from build123d import *

# Parameters (mm, degrees)
F1_DEPTH = 1.8542
F2_W     = 1.143
F2_H     = 2.4384
F3_DEPTH = 25.4


with BuildPart() as f1:
    # F0 (on Front) → F1 (new body, symmetric)
    with BuildSketch(Plane.XZ):
        Polygon((-6.975146, 2.699733), (-0.1143, 0), (-0.1143, -16.9164), (0.290897, -18.905481), (0.514896, -18.85985), (0.1143, -16.9164), (0.1143, 0), (0.1143, 0.155708), (-6.89144, 2.912456), align=None)
    extrude(amount=F1_DEPTH, both=True)

    # F2 (on face) → F3 (cut)
    with BuildSketch(Plane(origin=(-0.1143, 0, 0), x_dir=(0, -1, 0), z_dir=(-1, 0, 0))):
        with BuildLine():
            Line((-1.8542, -11.176), (-1.8542, -8.636))
            ThreePointArc((-1.8542, -8.636), (-3.1242, -9.906), (-1.8542, -11.176))
        make_face()
        with BuildLine():
            ThreePointArc((-0.5842, -9.906), (-0.956174, -9.007974), (-1.8542, -8.636))
            Line((-1.8542, -8.636), (-1.8542, -11.176))
            ThreePointArc((-1.8542, -11.176), (-0.956174, -10.804026), (-0.5842, -9.906))
        make_face()
        with BuildLine():
            ThreePointArc((3.1242, -9.906), (2.752226, -9.007974), (1.8542, -8.636))
            Line((1.8542, -8.636), (1.8542, -11.176))
            ThreePointArc((1.8542, -11.176), (2.752226, -10.804026), (3.1242, -9.906))
        make_face()
        with BuildLine():
            Line((1.8542, -11.176), (1.8542, -8.636))
            ThreePointArc((1.8542, -8.636), (0.5842, -9.906), (1.8542, -11.176))
        make_face()
        with Locations((-1.2827, -3.7592)):
            Rectangle(F2_W, F2_H)
    extrude(amount=-F3_DEPTH, mode=Mode.SUBTRACT)


solid = f1.part
Geometry: final body of the model. Coordinates: model frame, mm. A direction names the side the tool comes from. Give positions to 0.01 mm unless a question says otherwise; leave off trailing zeros. Order: outer loops, then holes, each group sorted by start corner. A loop starts at its lowest first (then second) coordinate and runs counter-clockwise, first axis right, second up. Notation, with made-up numbers: (27, 28) - (71, 28) arc R36 ccw to (71, 66) - close; hole circle Ø4 at (-29.75, -24.5). An arc over 180 degrees is marked (long way). Use CSV: the item, a comma, the result in double quotes.
1. Contact query for flat-ended pins moving along their axis: pin 1 (1.5 mm diameter, centred on x = -4, y = 0, fed in from +Z); pin 2 (1.1 mm diameter, centred on y = -0.5, z = -9, fed in from +X). Output: stop coordinate, or through.
Answers below:
pin 1,"z = 2.07"
pin 2,"x = 0.11"
2. Material intervals for line 1 along X through (y, z) = (0.75, -8.5); line 2 along Z through (x, y) = (-4.5, 1.45); line 3 along Z through (x, y) = (-6, 1.4), sorted ascending. Write a range as from..to.
Answers below:
line 1,"-0.11..0.11"
line 2,"1.73..1.97"
line 3,"2.32..2.56"
3. Section query A-A (y = -1.55). Output: boundary loops of the cut face in (x, z), plus the area to 3 significant figures.
Answers below:
outline,"(-6.98, 2.7) - (-0.11, 0) - (-0.11, -8.67) - (0.11, -8.67) - (0.11, 0.16) - (-6.89, 2.91) - close; (-0.11, -16.92) - (0.29, -18.91) - (0.51, -18.86) - (0.11, -16.92) - (0.11, -11.14) - (-0.11, -11.14) - close"
area,"5.48 mm2"
4. Section query B-B (y = 0.3). Output: boundary loops of the cut face in (x, z), plus the area to 3 significant figures.
Answers below:
outline,"(-6.98, 2.7) - (-0.11, 0) - (-0.11, -16.92) - (0.29, -18.91) - (0.51, -18.86) - (0.11, -16.92) - (0.11, 0.16) - (-6.89, 2.91) - close"
area,"6.04 mm2"
5. Access query for faces 1 (the face through (0.114, 0, -8)), 2 (the face through (-0.114, 0, -8)). Directions: +Z, -Z, +X, -X, +Y, -Y. A direction counts if a zero-diameter tool reaches every point of the face in a straight line with its end or side. Return the directions, or none.
Answers below:
face 1,"+Z, +X, +Y, -Y"
face 2,"-Z, -X, +Y, -Y"
6. Section query C-C (y = 1.65). Output: boundary loops of the cut face in (x, z).
Answers below:
outline,"(-6.98, 2.7) - (-0.11, 0) - (-0.11, -2.54) - (0.11, -2.54) - (0.11, 0.16) - (-6.89, 2.91) - close; (-0.11, -16.92) - (0.29, -18.91) - (0.51, -18.86) - (0.11, -16.92) - (0.11, -11.16) - (-0.11, -11.16) - close; (-0.11, -8.65) - (0.11, -8.65) - (0.11, -4.98) - (-0.11, -4.98) - close"
7. Section query D-D (z = -3.25). Output: boundary loops of the cut face in (x, y), plus the area to 3 significant figures.
Answers below:
outline,"(-0.11, -1.85) - (0.11, -1.85) - (0.11, 0.71) - (-0.11, 0.71) - close"
area,"0.586 mm2"
